Read the model definition and answer for the solid it produces. Units are mm, in the model's axes. A direction names the side the tool comes from. Round coordinates to 2 decimals unless told otherwise and drop trailing zeros. Write each loop counter-clockwise with the first axis right and the second up, starting at its lowest first coordinate (ties: lowest second). Pieces come first, ordered by that corner, then holes. Notation, with made-up numbers: (65.5, 1) - (121.5, 1) arc R27 ccw to (121.5, 36) - close; hole circle Ø10 at (-6.5, -11). An arc over 180 degrees is marked (long way). Use one line per item in the form item = value. Start each with the question number.
1) For faces 1 (the face through (-21.016, -12.325, 48.331)), 2 (the face through (-18.51, -12.32, 29.15)), determine the directions among +Z, -Z, +X, -X, +Y, -Y from which every point of the face is accessible in a straight line to the end or side of a thin tool.
2) Each of these flat-tipped pins is pushed along its axis until it touches: pin 1 (8 mm diameter, centred on y = -4.5, z = 37, fed in from -X); pin 2 (3 mm diameter, centred on x = -22.5, y = -8.5, fed in from +Z); pin 3 (10 mm diameter, centred on y = -12.5, z = 15.5, fed in from +X). Where does it stop, or does it pass through?
3) The part is cut by section C-C, the plane y = -18.5. Give the vertices of the cut face in (x, z), plus the area to 3 significant figures.
4) The part is cut by section D-D, the plane z = 24. Give the vertices of the cut face in (x, y).
5) Consider line 1 along X through (y, z) = (-20.5, -1.5); line 2 along Z through (x, y) = (-30, -16); line 3 along Z through (x, y) = (-32.5, -10.25). Determine where each line is inside the solid, lowest interval first. Write a range as from..to.
6) The part is cut by section B-B, the plane z = 65. Give the vertices of the cut face in (x, y), plus the area to 3 significant figures.
7) For a pull along Z with two mould halves and no side action, classify faces 3 (the face through (-30.06, -12.32, -1.22)), 4 (the face through (-31.663, -12.325, -3.851)), 5 (the face through (-28.4, -12.3, 70)) as released by +Z, released by -Z, zero draft, split by the parting line, or undercut.
8) The part is cut by section A-A, the plane x = -32. Give the vertices of the cut face in (y, z).
from build123d import *

# Parameters (mm, degrees)
F0_R     = 2
F1_DEPTH = 25


with BuildPart() as f1:
    # F0 (on Front) → F1 (new body)
    with BuildSketch(Plane.XZ):
        with BuildLine():
            ThreePointArc((-3.313569, -3.996799), (-7.473569, 0), (-3.313569, 3.996799))
            Line((-3.313569, 3.996799), (-16.919591, 4.541475))
            ThreePointArc((-16.919591, 4.541475), (-20.602202, 6.387025), (-21.649657, 10.370807))
            Line((-21.649657, 10.370807), (-18.613436, 28.333333))
            ThreePointArc((-18.613436, 28.333333), (-28.473569, 20), (-38.333702, 28.333333))
            Line((-38.333702, 28.333333), (-33.403636, -0.833333))
            ThreePointArc((-33.403636, -0.833333), (-28.8917, 4.982486), (-23.473569, 0))
            ThreePointArc((-23.473569, 0), (-24.868018, -3.464102), (-28.273569, -4.995998))
            Line((-28.273569, -4.995998), (-3.313569, -3.996799))
        make_face()
        with BuildLine():
            ThreePointArc((-33.403636, -0.833333), (-31.624018, -3.882612), (-28.273569, -4.995998))
            ThreePointArc((-28.273569, -4.995998), (-24.868018, -3.464102), (-23.473569, 0))
            ThreePointArc((-23.473569, 0), (-28.8917, 4.982486), (-33.403636, -0.833333))
        make_face()
        with Locations((-28.473569, 0)):
            Circle(F0_R, mode=Mode.SUBTRACT)
        with BuildLine():
            ThreePointArc((-3.313569, -3.996799), (-0.589128, -2.771281), (0.526431, 0))
            ThreePointArc((0.526431, 0), (-0.589128, 2.771281), (-3.313569, 3.996799))
            ThreePointArc((-3.313569, 3.996799), (-7.473569, 0), (-3.313569, -3.996799))
        make_face()
        with Locations((-3.473569, 0)):
            Circle(F0_R, mode=Mode.SUBTRACT)
        with BuildLine():
            ThreePointArc((-38.333702, 28.333333), (-28.473569, 20), (-18.613436, 28.333333))
            ThreePointArc((-18.613436, 28.333333), (-18.508597, 29.163737), (-18.473569, 30))
            ThreePointArc((-18.473569, 30), (-18.499244, 30.716124), (-18.576136, 31.428571))
            ThreePointArc((-18.576136, 31.428571), (-28.473569, 40), (-38.371002, 31.428571))
            ThreePointArc((-38.371002, 31.428571), (-38.472843, 29.8795), (-38.333702, 28.333333))
        make_face()
        with Locations((-28.473569, 30)):
            Circle(F0_R, mode=Mode.SUBTRACT)
        with BuildLine():
            Line((-33.422286, 65.714286), (-38.371002, 31.428571))
            ThreePointArc((-38.371002, 31.428571), (-28.473569, 40), (-18.576136, 31.428571))
            Line((-18.576136, 31.428571), (-23.524852, 65.714286))
            ThreePointArc((-23.524852, 65.714286), (-23.486406, 65.358062), (-23.473569, 65))
            ThreePointArc((-23.473569, 65), (-28.831631, 60.012837), (-33.422286, 65.714286))
        make_face()
        with Locations((-31.536311, 54.071311)):
            Circle(F0_R, mode=Mode.SUBTRACT)
        with BuildLine():
            ThreePointArc((-23.524852, 65.714286), (-28.473569, 70), (-33.422286, 65.714286))
            ThreePointArc((-33.422286, 65.714286), (-28.831631, 60.012837), (-23.473569, 65))
            ThreePointArc((-23.473569, 65), (-23.486406, 65.358062), (-23.524852, 65.714286))
        make_face()
        with Locations((-28.473569, 65)):
            Circle(F0_R, mode=Mode.SUBTRACT)
    extrude(amount=F1_DEPTH)


solid = f1.part
Geometry results:
q1.face_1 = +Z, +X, +Y, -Y
q1.face_2 = +X, +Y, -Y
q2.pin_1 = -38.14
q2.pin_2 = 67.23
q2.pin_3 = -19.94
q3.outline = (-38.37, 31.43) arc R10 ccw to (-38.33, 28.33) - (-33.4, -0.83) arc R5 ccw to (-28.27, -5) - (-3.31, -4) arc R4 ccw to (0.53, 0) arc R4 ccw to (-3.31, 4) - (-16.92, 4.54) arc R5 cw to (-21.65, 10.37) - (-18.61, 28.33) arc R10 ccw to (-18.47, 30) arc R10 ccw to (-18.58, 31.43) - (-23.52, 65.71) arc R5 ccw to (-33.42, 65.71) - close; hole circle Ø4 at (-31.54, 54.07); hole circle Ø4 at (-28.47, 0); hole circle Ø4 at (-28.47, 30); hole circle Ø4 at (-28.47, 65); hole circle Ø4 at (-3.47, 0)
q3.area = 1,210 mm2
q4.outline = (-37.6, -25) - (-19.35, -25) - (-19.35, 0) - (-37.6, 0) - close
q5.line_1 = -33.24..-29.8, -27.15..-4.8, -2.15..0.23
q5.line_2 = -4.76..-1.29, 1.29..28.71, 31.29..52.79, 55.35..63.71, 66.29..69.76
q5.line_3 = -2.96..52.32, 55.82..67.96
q6.outline = (-33.53, -25) - (-30.47, -25) - (-30.47, 0) - (-33.53, 0) - close; (-26.47, -25) - (-23.42, -25) - (-23.42, 0) - (-26.47, 0) - close
q6.area = 153 mm2
q7.face_3 = undercut
q7.face_4 = released by -Z
q7.face_5 = released by +Z
q8.outline = (-25, -3.54) - (0, -3.54) - (0, 52.13) - (-25, 52.13) - close; (-25, 56.02) - (0, 56.02) - (0, 68.54) - (-25, 68.54) - close
